Model file for the job. Use its own axes, mm. A direction names the side the tool comes from. Coordinates: 2 decimals unless noted, no trailing zeros. Write each loop counter-clockwise with the first axis right and the second up, starting at its lowest first coordinate (ties: lowest second). Pieces come first, ordered by that corner, then holes. Notation, with made-up numbers: (61.5, 61) -> (81.5, 61) arc R18 ccw to (81.5, 92) -> close; hole circle Ø9 at (34.25, 15). An arc over 180 degrees is marked (long way). Answer as a JSON object with one key per item and string values. Group by question number.
from build123d import *

# Parameters (mm, degrees)
F0_R      = 22.5
F1_DEPTH  = 21
F3_DEPTH  = 21
F6_DEPTH  = 9
F4_R      = 3.5
F7_DEPTH  = 12
F8_DEPTH  = 20
F9_DEPTH  = 9
F11_DEPTH = 20
F10_R     = 3.5
F12_DEPTH = 12
F2_R      = 1.5
F13_DEPTH = 21.001


with BuildPart() as f1:
    # F0 (on Front) → F1 (new body)
    with BuildSketch(Plane.XZ):
        Circle(F0_R)
    extrude(amount=F1_DEPTH)

    # F2 (on face) → F3 (join)
    with BuildSketch(Plane.XZ.offset(21)):
        with BuildLine():
            Line((22, 22.5), (10, 22.5))
            Line((10, 22.5), (10, 20.1556443707))
            ThreePointArc((10, 20.1556443707), (10.1541802531, 20.0784118741), (10.307764064, 20))
            Line((10.307764064, 20), (22, 20))
            Line((22, 20), (22, 22.5))
        make_face()
        with BuildLine():
            ThreePointArc((10.307764064, -20), (10.1541802531, -20.0784118741), (10, -20.1556443707))
            Line((10, -20.1556443707), (10, -22.5))
            Line((10, -22.5), (22, -22.5))
            Line((22, -22.5), (22, -20))
            Line((22, -20), (10.307764064, -20))
        make_face()
        with BuildLine():
            ThreePointArc((10.307764064, 20), (10.1541802531, 20.0784118741), (10, 20.1556443707))
            Line((10, 20.1556443707), (10, 20))
            Line((10, 20), (10.307764064, 20))
        make_face()
        with BuildLine():
            Line((10, -20), (10, -20.1556443707))
            ThreePointArc((10, -20.1556443707), (10.1541802531, -20.0784118741), (10.307764064, -20))
            Line((10.307764064, -20), (10, -20))
        make_face()
    extrude(amount=-F3_DEPTH)

    # F5 (on face) → F6 (cut)
    with BuildSketch(Plane(origin=(0, 0, 0), x_dir=(-1, 0, 0), z_dir=(0, 1, 0))):
        Polygon((-10.307764064, 20), (-10, 20.1556443707), (-10, 22.5), (-22, 22.5), (-22, 20), align=None)
    extrude(amount=-F6_DEPTH, mode=Mode.SUBTRACT)

    # F4 (on face) → F7 (join)
    with BuildSketch(Plane.XY.offset(22.5)):
        with Locations((16, -15)):
            Circle(F4_R)
    extrude(amount=F7_DEPTH)

    # F8 (add): a face of the model
    f8_faces = [f1.faces().sort_by_distance(p)[0] for p in [
        (16.153882032, -15, 20),
    ]]
    extrude(f8_faces, amount=F8_DEPTH)

    # F2 (on face) → F9 (cut)
    with BuildSketch(Plane.XZ.offset(21)):
        with BuildLine():
            ThreePointArc((10.307764064, -20), (10.1541802531, -20.0784118741), (10, -20.1556443707))
            Line((10, -20.1556443707), (10, -22.5))
            Line((10, -22.5), (22, -22.5))
            Line((22, -22.5), (22, -20))
            Line((22, -20), (10.307764064, -20))
        make_face()
    extrude(amount=-F9_DEPTH, mode=Mode.SUBTRACT)

    # F11 (add): a face of the model
    f11_faces = [f1.faces().sort_by_distance(p)[0] for p in [
        (16.153882032, -6, -20),
    ]]
    extrude(f11_faces, amount=F11_DEPTH)

    # F10 (on face) → F12 (join)
    with BuildSketch(Plane(origin=(0, 0, -22.5), x_dir=(1, 0, 0), z_dir=(0, 0, -1))):
        with Locations((16, 6)):
            Circle(F10_R)
    extrude(amount=F12_DEPTH)

    # F2 (on face) → F13 (cut, through all)
    with BuildSketch(Plane.XZ.offset(21)):
        with Locations((8.1317279836, -8.1317279836)):
            Circle(F2_R)
        with Locations((-8.1317279836, 8.1317279836)):
            Circle(F2_R)
    extrude(amount=-F13_DEPTH, mode=Mode.SUBTRACT)


solid = f1.part
(1) Cut at A-A on y = -6. List the corners of the cut face in (x, z).
(2) Pull direction X, two halves, no side cores. Call faces 6 (the face through (17.615, -18.105, 28.416)), 7 (the face through (10, -15, 21)), 8 (the face through (22, -15, 14)), 9 (the face through (-6.746, -10.647, 7.557)): released by +X, released by -X, zero draft, split by the parting line, or undercut.
(3) Cut at D-D on x = 14.5. List the corners of the cut face in (y, z), plus the area to 3 significant figures.
(4) 3-axis set-ups, long thin cutter, end or side, ignore diameter. For faces 1 (the face through (22, -6, -14)), 2 (the face through (13, -12, 22.5)), 3 (the face through (19, -9, -22.5)), 4 (the face through (17, -12, -18)), 5 (the face through (17, -9, 18)): which of +Z, -Z, +X, -X, +Y, -Y reach the whole face in a straight line?
(5) Cut at B-B on x = 0. List the corners of the cut face in (y, z).
(6) Pin check, flat tips, straight feed: pin 1 (2 mm diameter, centred on x = 1.5, y = -13, fed in from +Z); pin 2 (3.5 mm diameter, centred on x = 8.13, z = -8.13, fed in from +Y); pin 3 (3.5 mm diameter, centred on y = -3, z = -10, fed in from +X); pin 4 (1 mm diameter, centred on x = -4.5, y = -7.5, fed in from -Z). Stop position of each tip, or through.
(7) Wall check: probe 1 along Z at (x, y) = (7, -7); probe 2 along Z at (x, y) = (-10, -13.25); probe 3 along Y at (x, z) = (20, -19). Give the ranges that are in metal, low to high.
(8) Cut at C-C on z = -25. List the corners of the cut face in (x, y).
Results found:
{
 "1": {"outline": "(10, -22.5) -> (12.5, -22.5) -> (12.5, -34.5) -> (19.5, -34.5) -> (19.5, -22.5) -> (22, -22.5) -> (22, -4.72) arc R22.5 ccw to (10.31, 20) -> (10, 20.16) arc R22.5 ccw (long way) to (10, -20.16) -> close; hole circle Ø3 at (-8.13, 8.13); hole circle Ø3 at (8.13, -8.13)"},
 "2": {"face 6": "split by the parting line", "face 7": "undercut", "face 8": "released by +X", "face 9": "undercut"},
 "3": {"outline": "(-21, -17.2) -> (-12, -17.2) -> (-12, -22.5) -> (-9.16, -22.5) -> (-9.16, -34.5) -> (-2.84, -34.5) -> (-2.84, -22.5) -> (0, -22.5) -> (0, 17.2) -> (-9, 17.2) -> (-9, 22.5) -> (-11.84, 22.5) -> (-11.84, 34.5) -> (-18.16, 34.5) -> (-18.16, 22.5) -> (-21, 22.5) -> close", "area": "1,000 mm²"},
 "4": {"face 1": "-Z, +X, +Y, -Y", "face 2": "+Z", "face 3": "-Z", "face 4": "-Z, +X, -Y", "face 5": "+Z, +X, +Y"},
 "5": {"outline": "(-21, -22.5) -> (0, -22.5) -> (0, 22.5) -> (-21, 22.5) -> close"},
 "6": {"pin 1": "stops at z = 22.49", "pin 2": "stops at y = 0", "pin 3": "stops at x = 22", "pin 4": "stops at z = -22.14"},
 "7": {"probe 1": "z = -21.38 to -9.12, -7.15 to 21.38", "probe 2": "z = -20.16 to 20.16", "probe 3": "y = -12 to 0"},
 "8": {"outline": "circle Ø7 at (16, -6)"}
}
